The listing builds one solid part. Answer for the finished solid, in the listing's coordinates (mm). Face numbers are marked on the shaded views. A direction names the side the tool comes from. Give positions to 0.01 mm unless a question says otherwise; leave off trailing zeros. Order: outer loops, then holes, each group sorted by start corner. A loop starts at its lowest first (then second) coordinate and runs counter-clockwise, first axis right, second up. Notation, with made-up numbers: (47, -32) - (102, -32) arc R17 ccw to (102, -10) - close; hole circle Ø3 at (-19, 78.25). An arc over 180 degrees is marked (long way). Answer as CSV lines item,"result". Start each with the question number.
1. Section A-A on x = 46 is taken. Give the vertices of the cut face in (y, z), and give its area (3 significant figures).
2. Consider line 1 along Z through (x, y) = (0.65, 160); line 2 along X through (y, z) = (71, 0.8); line 3 along Y through (x, z) = (15, 0.65). Determine where each line is inside the solid, lowest interval first. Write a range as [from, to].
3. Section C-C on y = 91 is taken. Give the vertices of the cut face in (x, z).
4. Section D-D on y = 71 is taken. Give the vertices of the cut face in (x, z).
5. Flat-ended cylindrical pins translate along their axes: pin 1 (7 mm diameter, centred on y = 8, z = 50, fed in from +X); pin 2 (8 mm diameter, centred on x = 40, y = 101, fed in from +Z). Find the tip coordinate at first contact, or state that the pin passes through.
6. Section B-B on z = 50 is taken. Give the vertices of the cut face in (x, y), and give its area (3 significant figures).
7. Which of the six approach directions +Z, -Z, +X, -X, +Y, -Y give full straight-line access (tool end or side, diameter ignored) to the marked faces 1 and 2?
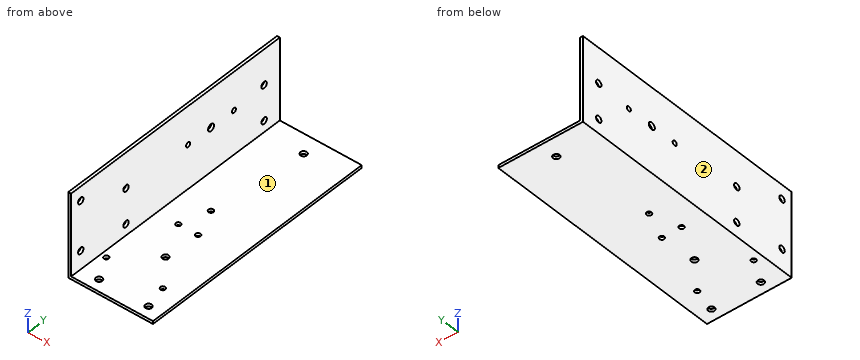
from build123d import *

# Parameters (mm, degrees)
LINEAR_AUSTRAGEN_D_NN1_DEPTH     = 173
DURCHGANGSLOCH_F_R_M41_D         = 4.5
DURCHGANGSLOCH_F_R_M42_D         = 4.5
DURCHGANGSLOCH_F_R_M43_D         = 4.5
DURCHGANGSLOCH_F_R_M31_D         = 3.4
F_5_0_5_DURCHMESSER_BOHRUNG1_D   = 5
DURCHGANGSLOCH_F_R_M32_D         = 3.4
DURCHGANGSLOCH_F_R_M33_D         = 3.4
F_3_5_3_5_DURCHMESSER_BOHRUNG1_D = 3.5


with BuildPart() as part:
    # Skizze1 → Linear-Austragen-Dünn1 (new body)
    with BuildSketch(Plane(origin=(0, 0, 0), x_dir=(1, 0, 0), z_dir=(0, 1, 0))):
        Polygon((60, 0), (0, 0), (0, -60), (2, -60), (2, -2), (60, -2), align=None)
    extrude(amount=LINEAR_AUSTRAGEN_D_NN1_DEPTH)

    # Durchgangsloch für M41 (through all)
    with Locations(Plane.ZY):
        with Locations((35, 160), (10, 160)):
            Hole(DURCHGANGSLOCH_F_R_M41_D / 2)

    # Durchgangsloch für M42 (through all)
    with Locations(Plane.ZY):
        with Locations((35, 45.5), (10, 45.5), (50, 8), (15, 8)):
            Hole(DURCHGANGSLOCH_F_R_M42_D / 2)

    # Durchgangsloch für M43 (through all)
    with Locations(Plane(origin=(0, 0, 0), x_dir=(-1, 0, 0), z_dir=(0, 0, -1))):
        with Locations((-30, 45.5), (-50, 8), (-15, 8), (-30, 160)):
            Hole(DURCHGANGSLOCH_F_R_M43_D / 2)

    # Durchgangsloch für M31 (through all)
    with Locations(Plane.ZY):
        with Locations((33, 97), (33, 135)):
            Hole(DURCHGANGSLOCH_F_R_M31_D / 2)

    # Ø5.0 (5) Durchmesser Bohrung1 (through all)
    with Locations(Plane.ZY):
        with Locations((33, 116)):
            Hole(F_5_0_5_DURCHMESSER_BOHRUNG1_D / 2)

    # Durchgangsloch für M32 (through all)
    with Locations(Plane(origin=(0, 0, 0), x_dir=(-1, 0, 0), z_dir=(0, 0, -1))):
        with Locations((-31.299999687, 71), (-17.299999687, 71)):
            Hole(DURCHGANGSLOCH_F_R_M32_D / 2)

    # Durchgangsloch für M33 (through all)
    with Locations(Plane(origin=(0, 0, 0), x_dir=(-1, 0, 0), z_dir=(0, 0, -1))):
        with Locations((-46, 24.5), (-6, 24.5)):
            Hole(DURCHGANGSLOCH_F_R_M33_D / 2)

    # Ø3.5 (3.5) Durchmesser Bohrung1 (through all)
    with Locations(Plane(origin=(0, 0, 0), x_dir=(-1, 0, 0), z_dir=(0, 0, -1))):
        with Locations((-23.299999687, 91)):
            Hole(F_3_5_3_5_DURCHMESSER_BOHRUNG1_D / 2)


solid = part.part
Checks:
1,outline,"(0, 0) - (22.8, 0) - (22.8, 2) - (0, 2) - close; (26.2, 0) - (173, 0) - (173, 2) - (26.2, 2) - close"
1,area,"339 mm²"
2,line 1,"z = [0, 7.75], [12.25, 32.75], [37.25, 60]"
2,line 2,"x = [0, 15.6], [19, 29.6], [33, 60]"
2,line 3,"y = [0, 5.75], [10.25, 173]"
3,outline,"(0, 0) - (21.55, 0) - (21.55, 2) - (2, 2) - (2, 60) - (0, 60) - close; (25.05, 0) - (60, 0) - (60, 2) - (25.05, 2) - close"
4,outline,"(0, 0) - (15.6, 0) - (15.6, 2) - (2, 2) - (2, 60) - (0, 60) - close; (19, 0) - (29.6, 0) - (29.6, 2) - (19, 2) - close; (33, 0) - (60, 0) - (60, 2) - (33, 2) - close"
5,pin 1,"stops at x = 2"
5,pin 2,"stops at z = 2"
6,outline,"(0, 0) - (2, 0) - (2, 5.75) - (0, 5.75) - close; (0, 10.25) - (2, 10.25) - (2, 173) - (0, 173) - close"
6,area,"337 mm²"
7,face 1,"+Z, +X, +Y, -Y"
7,face 2,"+Z, -Z, -X, +Y, -Y"
